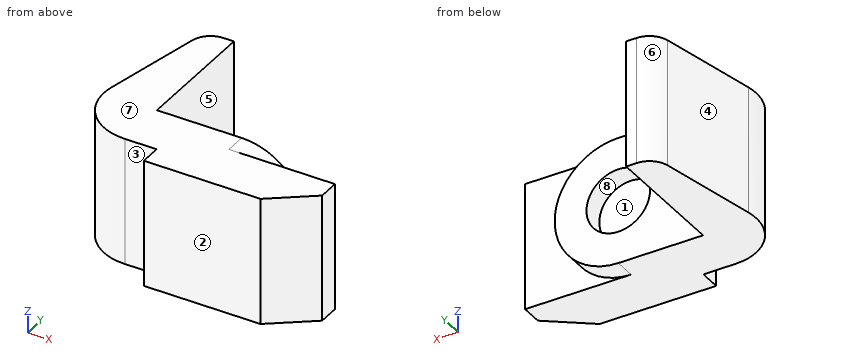
```python
from build123d import *

# Parameters (mm, degrees)
BOSS_EXTRUDE1_DEPTH = 76.2
SKETCH3_R           = 38.1
BOSS_EXTRUDE2_DEPTH = 12.7
SKETCH4_R           = 19.05
CUT_EXTRUDE1_DEPTH  = 12.7


with BuildPart() as part:
    # Sketch1 → Boss-Extrude1 (new body)
    with BuildSketch(Plane.XY):
        with BuildLine():
            Line((0, 0), (69.85, 0))
            Line((69.85, 0), (95.25, 19.05))
            Line((95.25, 19.05), (95.25, 31.75))
            Line((95.25, 31.75), (31.75, 31.75))
            Line((31.75, 31.75), (31.75, 44.45))
            Line((31.75, 44.45), (-19.05, 44.45))
            Line((-19.05, 44.45), (-19.05, 120.65))
            Line((-19.05, 120.65), (-25.4, 120.65))
            ThreePointArc((-25.4, 120.65), (-33.421823369, 117.795829058), (-37.838031752, 110.516196825))
            Line((-37.838031752, 110.516196825), (-50.145079379, 50.865492062))
            ThreePointArc((-50.145079379, 50.865492062), (-43.664572645, 24.395441578), (-19.05, 12.7))
            Line((-19.05, 12.7), (0, 12.7))
            Line((0, 12.7), (0, 0))
        make_face()
    extrude(amount=BOSS_EXTRUDE1_DEPTH)

    # Sketch3 → Boss-Extrude2 (add)
    with BuildSketch(Plane(origin=(0, 31.75, 0), x_dir=(1, 0, 0), z_dir=(0, 1, 0))):
        with Locations((31.75, -38.1)):
            Circle(SKETCH3_R)
    extrude(amount=BOSS_EXTRUDE2_DEPTH)

    # Sketch4 → Cut-Extrude1 (cut)
    with BuildSketch(Plane(origin=(0, 44.45, 0), x_dir=(1, 0, 0), z_dir=(0, 1, 0))):
        with Locations(Location((31.75, -38.1, 0), (0, 0, 180))):
            Circle(SKETCH4_R)
    extrude(amount=-CUT_EXTRUDE1_DEPTH, mode=Mode.SUBTRACT)


solid = part.part
```
Geometry: final body of the model. Coordinates: model frame, mm. Face numbers are marked on the shaded views. A direction names the side the tool comes from. Round coordinates to 2 decimals unless told otherwise and drop trailing zeros. Order: outer loops, then holes, each group sorted by start corner. A loop starts at its lowest first (then second) coordinate and runs counter-clockwise, first axis right, second up. Notation, with made-up numbers: (53, 79) -> (111, 79) arc R27 cw to (111, 96) -> close; hole circle Ø3 at (43.5, -6.75). An arc over 180 degrees is marked (long way). Use one line per item in the form item = value.
(1) First-contact query: pin 1 Ø3 at (y, z) = (39, 51.5) entering from +X; pin 2 Ø1 at (x, z) = (23.5, 13) entering from +Y; pin 3 Ø5 at (y, z) = (16.5, 18.5) entering from +X; pin 4 Ø23 at (x, z) = (31.75, 38.1) entering from -Y. Flat tips, straight axial feed; report the tip coordinate or a pass-through.
Results list:
pin_1 = 67.94
pin_2 = 44.45
pin_3 = 95.18
pin_4 = 0
(2) Section C-C on y = 30. Return loops of the section in (x, z), and give its area (3 significant figures).
Results list:
outline = (-47.32, 0) -> (95.25, 0) -> (95.25, 76.2) -> (-47.32, 76.2) -> close
area = 10,900 mm^2
(3) Access query for the marked faces 1, 2, 3, 4 and 5. Directions: +Z, -Z, +X, -X, +Y, -Y. A direction counts if a zero-diameter tool reaches every point of the face in a straight line with its end or side. Return the directions, or none.
Results list:
face_1 = +Y
face_2 = +Z, -Z, +X, -X, -Y
face_3 = +Z, -Z, -X, -Y
face_4 = +Z, -Z, -X, +Y
face_5 = +Z, -Z, +X, +Y
(4) Ray query, probe 1 along Z at (x, y) = (31.75, 40.5); probe 2 along Y at (x, z) = (-4.5, 43); probe 3 along X at (y, z) = (35, 45.5). Return the intervals inside material, ascending. Write a range as [from, to].
Results list:
probe_1 = [0, 19.05], [57.15, 76.2]
probe_2 = [12.7, 44.45]
probe_3 = [-49.36, 14.2], [49.3, 69.12]
(5) Section D-D on z = 55. Return loops of the section in (x, y), and give its area (3 significant figures).
Results list:
outline = (-50.15, 50.87) arc R31.75 ccw to (-19.05, 12.7) -> (0, 12.7) -> (0, 0) -> (69.85, 0) -> (95.25, 19.05) -> (95.25, 31.75) -> (65.9, 31.75) -> (65.9, 44.45) -> (40.54, 44.45) -> (40.54, 31.75) -> (22.96, 31.75) -> (22.96, 44.45) -> (-19.05, 44.45) -> (-19.05, 120.65) -> (-25.4, 120.65) arc R12.7 ccw to (-37.84, 110.52) -> close
area = 6,640 mm^2
(6) Section A-A on z = 38.1. Return loops of the section in (x, y).
Results list:
outline = (-50.15, 50.87) arc R31.75 ccw to (-19.05, 12.7) -> (0, 12.7) -> (0, 0) -> (69.85, 0) -> (95.25, 19.05) -> (95.25, 31.75) -> (69.85, 31.75) -> (69.85, 44.45) -> (50.8, 44.45) -> (50.8, 31.75) -> (12.7, 31.75) -> (12.7, 44.45) -> (-19.05, 44.45) -> (-19.05, 120.65) -> (-25.4, 120.65) arc R12.7 ccw to (-37.84, 110.52) -> close
(7) Section B-B on x = 54.5. Return loops of the section in (y, z).
Results list:
outline = (0, 0) -> (31.75, 0) -> (31.75, 7.54) -> (44.45, 7.54) -> (44.45, 68.66) -> (31.75, 68.66) -> (31.75, 76.2) -> (0, 76.2) -> close
(8) Draft query along Z for the marked faces 6, 7 and 8. Return one class per face: pulls with the +Z half, pulls with the -Z half, needs draft (parallel to the pull), parting line crosses it, or undercut.
Results list:
face_6 = needs draft
face_7 = pulls with the +Z half
face_8 = undercut
